```python
from build123d import *

# Parameters (mm, degrees)
BOSS_EXTRUDE1_DEPTH = 3
SKETCH1_9_R         = 1.5
SKETCH1_9_W         = 3
SKETCH1_9_H         = 3.9
SKETCH1_9_W_2       = 7.8
SKETCH1_9_H_2       = 3
BOSS_EXTRUDE2_DEPTH = 27
SKETCH2_W           = 22
SKETCH2_H           = 3.9
BOSS_EXTRUDE3_DEPTH = 2.5
CUT_EXTRUDE1_REACH  = 183.139
SKETCH6_R           = 1.95
SKETCH1_12_R        = 1.6
CUT_EXTRUDE7_DEPTH  = 105.877309271
SKETCH7_R           = 5
CUT_EXTRUDE8_DEPTH  = 10
FILLET1_R           = 3
FILLET2_R           = 3
CUT_EXTRUDE9_START  = -7.3
SKETCH8_W           = 11.4
SKETCH8_H           = 17.4
CUT_EXTRUDE9_DEPTH  = 33.4


with BuildPart() as part:
    # Sketch1 → Boss-Extrude1 (new body)
    with BuildSketch(Plane(origin=(0, 0, 0), x_dir=(1, 0, 0), z_dir=(0, 1, 0))):
        with BuildLine():
            ThreePointArc((-92, -22.5), (-86.142135624, -36.642135624), (-72, -42.5))
            Line((-72, -42.5), (72, -42.5))
            ThreePointArc((72, -42.5), (86.142135624, -36.642135624), (92, -22.5))
            Line((92, -22.5), (92, 34.5))
            Line((92, 34.5), (50, 34.5))
            Line((50, 34.5), (50, 42.5))
            Line((50, 42.5), (-50, 42.5))
            Line((-50, 42.5), (-50, 34.5))
            Line((-50, 34.5), (-92, 34.5))
            Line((-92, 34.5), (-92, -22.5))
        make_face()
    extrude(amount=BOSS_EXTRUDE1_DEPTH)

    # Sketch1<9> → Boss-Extrude2 (add)
    # profile 1 of 13: a face of its own
    with BuildSketch(Plane(origin=(0, 0, 0), x_dir=(1, 0, 0), z_dir=(0, 1, 0))):
        with BuildLine():
            ThreePointArc((-92, -22.5), (-86.142135624, -36.642135624), (-72, -42.5))
            Line((-72, -42.5), (72, -42.5))
            ThreePointArc((72, -42.5), (86.142135624, -36.642135624), (92, -22.5))
            Line((92, -22.5), (92, 34.5))
            Line((92, 34.5), (50, 34.5))
            Line((50, 34.5), (50, 42.5))
            Line((50, 42.5), (-50, 42.5))
            Line((-50, 42.5), (-50, 34.5))
            Line((-50, 34.5), (-92, 34.5))
            Line((-92, 34.5), (-92, -22.5))
        make_face()
        with Locations(Location((0, -39.5, 0), (0, 0, 270))):
            Circle(SKETCH1_9_R, mode=Mode.SUBTRACT)
        with Locations(Location((-89, 31.5, 0), (0, 0, 270))):
            Circle(SKETCH1_9_R, mode=Mode.SUBTRACT)
        with Locations(Location((-47, 39.5, 0), (0, 0, 270))):
            Circle(SKETCH1_9_R, mode=Mode.SUBTRACT)
        Polygon((-72, -36.5), (-86, -36.5), (-86, -22.5), (-86, 28.5), (-44, 28.5), (-44, 36.5), (44, 36.5), (44, 28.5), (86, 28.5), (86, -22.5), (86, -36.5), (72, -36.5), align=None, mode=Mode.SUBTRACT)
        with Locations(Location((89, 31.5, 0), (0, 0, 270))):
            Circle(SKETCH1_9_R, mode=Mode.SUBTRACT)
        with Locations(Location((47, 39.5, 0), (0, 0, 270))):
            Circle(SKETCH1_9_R, mode=Mode.SUBTRACT)
    # profile 2 of 13: a face of its own
    with BuildSketch(Plane(origin=(0, 0, 0), x_dir=(1, 0, 0), z_dir=(0, 1, 0))):
        Polygon((-57, 19.75), (-54, 19.75), (-54, 22.75), (-61.8, 22.75), (-61.8, 19.75), align=None)
    # profile 3 of 13: a face of its own
    with BuildSketch(Plane(origin=(0, 0, 0), x_dir=(1, 0, 0), z_dir=(0, 1, 0))):
        with Locations((-55.5, 17.8)):
            Rectangle(SKETCH1_9_W, SKETCH1_9_H)
    # profile 4 of 13: a face of its own
    with BuildSketch(Plane(origin=(0, 0, 0), x_dir=(1, 0, 0), z_dir=(0, 1, 0))):
        Polygon((-54, 12.85), (-54, 15.85), (-57, 15.85), (-79, 15.85), (-79, 12.85), align=None)
    # profile 5 of 13: a face of its own
    with BuildSketch(Plane(origin=(0, 0, 0), x_dir=(1, 0, 0), z_dir=(0, 1, 0))):
        Polygon((-82, 19.75), (-79, 19.75), (-74.2, 19.75), (-74.2, 22.75), (-82, 22.75), align=None)
    # profile 6 of 13: a face of its own
    with BuildSketch(Plane(origin=(0, 0, 0), x_dir=(1, 0, 0), z_dir=(0, 1, 0))):
        Polygon((-79, 12.85), (-79, 15.85), (-79, 19.75), (-82, 19.75), (-82, 12.85), align=None)
    # profile 7 of 13: a face of its own
    with BuildSketch(Plane(origin=(0, 0, 0), x_dir=(1, 0, 0), z_dir=(0, 1, 0))):
        with Locations((57.9, 21.25)):
            Rectangle(SKETCH1_9_W_2, SKETCH1_9_H_2)
    # profile 8 of 13: a face of its own
    with BuildSketch(Plane(origin=(0, 0, 0), x_dir=(1, 0, 0), z_dir=(0, 1, 0))):
        with Locations((55.5, 17.8)):
            Rectangle(SKETCH1_9_W, SKETCH1_9_H)
    # profile 9 of 13: a face of its own
    with BuildSketch(Plane(origin=(0, 0, 0), x_dir=(1, 0, 0), z_dir=(0, 1, 0))):
        Polygon((79, 15.85), (57, 15.85), (54, 15.85), (54, 12.85), (79, 12.85), align=None)
    # profile 10 of 13: a face of its own
    with BuildSketch(Plane(origin=(0, 0, 0), x_dir=(1, 0, 0), z_dir=(0, 1, 0))):
        with Locations((78.1, 21.25)):
            Rectangle(SKETCH1_9_W_2, SKETCH1_9_H_2)
    # profile 11 of 13: a face of its own
    with BuildSketch(Plane(origin=(0, 0, 0), x_dir=(1, 0, 0), z_dir=(0, 1, 0))):
        Polygon((79, 19.75), (79, 15.85), (79, 12.85), (82, 12.85), (82, 19.75), align=None)
    # profile 12 of 13: a face of its own
    with BuildSketch(Plane(origin=(0, 0, 0), x_dir=(1, 0, 0), z_dir=(0, 1, 0))):
        with BuildLine():
            Line((-86, -22.5), (-86, -36.5))
            Line((-86, -36.5), (-72, -36.5))
            ThreePointArc((-72, -36.5), (-81.899494937, -32.399494937), (-86, -22.5))
        make_face()
        with Locations(Location((-84.02081528, -34.52081528, 0), (0, 0, 270))):
            Circle(SKETCH1_9_R, mode=Mode.SUBTRACT)
    # profile 13 of 13: a face of its own
    with BuildSketch(Plane(origin=(0, 0, 0), x_dir=(1, 0, 0), z_dir=(0, 1, 0))):
        with BuildLine():
            ThreePointArc((86, -22.5), (81.899494937, -32.399494937), (72, -36.5))
            Line((72, -36.5), (86, -36.5))
            Line((86, -36.5), (86, -22.5))
        make_face()
        with Locations(Location((84.02081528, -34.52081528, 0), (0, 0, 270))):
            Circle(SKETCH1_9_R, mode=Mode.SUBTRACT)
    extrude(amount=BOSS_EXTRUDE2_DEPTH)

    # Sketch2 → Boss-Extrude3 (add)
    with BuildSketch(Plane(origin=(0, 3, 0), x_dir=(1, 0, 0), z_dir=(0, 1, 0))):
        with Locations((-68, 17.8)):
            Rectangle(SKETCH2_W, SKETCH2_H)
        with Locations((68, 17.8)):
            Rectangle(SKETCH2_W, SKETCH2_H)
    extrude(amount=BOSS_EXTRUDE3_DEPTH)

    # Cut-Extrude1: up to this face of the body (flat: up to its plane)
    cut_extrude1_end = Plane(part.part.faces().sort_by_distance((82, 15, -17.8))[0])
    # Sketch6 → Cut-Extrude1 (cut, up to the picked face)
    with BuildSketch(Plane.ZY.offset(82), mode=Mode.PRIVATE) as cut_extrude1_sk1:
        with Locations((-17.8, 16.5)):
            Circle(SKETCH6_R)
    cut_extrude1_tool1 = split(extrude(cut_extrude1_sk1.sketch, amount=-CUT_EXTRUDE1_REACH, mode=Mode.PRIVATE), bisect_by=cut_extrude1_end, keep=Keep.BOTH, mode=Mode.PRIVATE)
    add(cut_extrude1_tool1.solids().sort_by(Axis((-82, 16.5, -17.8), (1, 0, 0)))[0], mode=Mode.SUBTRACT)

    # Sketch1<12> → Cut-Extrude7 (cut, through all)
    with BuildSketch(Plane(origin=(0, 0, 0), x_dir=(1, 0, 0), z_dir=(0, 1, 0))):
        with Locations(Location((-64.4, -13.9, 0), (0, 0, 270))):
            Circle(SKETCH1_12_R)
        with Locations(Location((-37.6, -13.9, 0), (0, 0, 270))):
            Circle(SKETCH1_12_R)
        with Locations(Location((64.4, 5.9, 0), (0, 0, 270))):
            Circle(SKETCH1_12_R)
        with Locations(Location((37.6, 5.9, 0), (0, 0, 270))):
            Circle(SKETCH1_12_R)
        with Locations(Location((64.4, -13.9, 0), (0, 0, 270))):
            Circle(SKETCH1_12_R)
        with Locations(Location((37.6, -13.9, 0), (0, 0, 270))):
            Circle(SKETCH1_12_R)
        with Locations(Location((-64.4, 5.9, 0), (0, 0, 270))):
            Circle(SKETCH1_12_R)
        with Locations(Location((-37.6, 5.9, 0), (0, 0, 270))):
            Circle(SKETCH1_12_R)
    extrude(amount=CUT_EXTRUDE7_DEPTH, mode=Mode.SUBTRACT)

    # Sketch7 → Cut-Extrude8 (cut)
    with BuildSketch(Plane(origin=(0, 0, -42.5), x_dir=(-1, 0, 0), z_dir=(0, 0, -1))):
        with Locations((0, 15)):
            Circle(SKETCH7_R)
    extrude(amount=-CUT_EXTRUDE8_DEPTH, mode=Mode.SUBTRACT)

    # Fillet1
    fillet1_edges = [part.edges().sort_by_distance(p)[0] for p in [
        (-86, 15, -28.5),
        (-44, 15, -28.5),
        (-44, 15, -36.5),
        (44, 15, -36.5),
        (44, 15, -28.5),
        (-92, 13.5, -34.5),
        (-50, 13.5, -34.5),
        (-50, 13.5, -42.5),
        (50, 13.5, -42.5),
        (50, 13.5, -34.5),
        (92, 13.5, -34.5),
    ]]
    fillet(fillet1_edges, radius=FILLET1_R)

    # Fillet2
    fillet2_edges = [part.edges().sort_by_distance(p)[0] for p in [
        (54, 15, -22.75),
        (54, 15, -12.85),
        (82, 15, -12.85),
        (82, 15, -22.75),
        (-82, 15, -22.75),
        (-82, 15, -12.85),
        (-54, 15, -12.85),
        (-54, 15, -22.75),
    ]]
    fillet(fillet2_edges, radius=FILLET2_R - 0.0001)  # a hair under: the kernel refuses the full size

    # Sketch8 → Cut-Extrude9 (cut)
    with BuildSketch(Plane.ZY.offset(92).offset(CUT_EXTRUDE9_START)):
        with Locations((-31.1, 16.5)):
            Rectangle(SKETCH8_W, SKETCH8_H)
    cut_extrude9 = extrude(amount=-CUT_EXTRUDE9_DEPTH, mode=Mode.SUBTRACT)

    # Mirror1: Cut-Extrude9 across plane
    add(cut_extrude9.mirror(Plane(origin=(0, 0, 0), x_dir=(0, 0, 1), z_dir=(1, 0, 0))), mode=Mode.SUBTRACT)


solid = part.part
```
Work out the finished part from the listing and answer in its coordinate system (mm). A direction names the side the tool comes from. Round coordinates to 2 decimals unless told otherwise and drop trailing zeros. Write each loop counter-clockwise with the first axis right and the second up, starting at its lowest first coordinate (ties: lowest second). Pieces come first, ordered by that corner, then holes. Notation, with made-up numbers: (42.25, -13.5) -> (51.25, -13.5) arc R23 ccw to (51.25, 10.5) -> close; hole circle Ø10 at (11.5, 60). An arc over 180 degrees is marked (long way). Write each question's results on one line, items separated by ' | '.
Q1. Determine the mould class of faces 5 (the flat face through (79, 10, -18)), 6 (the flat face through (67.8, 27, -15.7)), 7 (the cylindrical face through (1.08, 10.12, -39.54)) for opening direction Y: released by +Y, released by -Y, zero draft, split by the parting line, or undercut.
Data:
face 5: zero draft | face 6: released by +Y | face 7: undercut
Q2. Flat-ended cylindrical pins translate along their axes: P1, Ø6, axis at x = -58, y = 5.5, coming from the -Z side; P2, Ø2.5, axis at x = 89, z = -31.5, coming from the +Y side. Find the tip coordinate at first contact, or state that the pin passes through.
Data:
P1: z = -34.5 | P2: y = 3
Q3. Section B-B, the plane y = 12.5 is taken. Give the number of separate pieces and of enclosed holes in the cut face, then the cut area to 3 significant figures.
Data:
separate pieces: 5 | enclosed holes: 7 | area: 2,780 mm^2
Q4. Straight lines are drawn through the part: line 1 along X through (y, z) = (13.25, -31.5); line 2 along X through (y, z) = (10, -18.5); line 3 along X through (y, z) = (2.05, 13.9). For each, find the intervals that lie inside material, in ascending order. Write a range as [from, to].
Data:
line 1: [-92, -90.5], [-87.5, -84.7], [-51.3, -44], [44, 51.3], [84.7, 87.5], [90.5, 92] | line 2: [-92, -86], [-82, -79], [-57, -54], [54, 57], [79, 82], [86, 92] | line 3: [-92, -66], [-62.8, -39.2], [-36, 36], [39.2, 62.8], [66, 92]
Q5. Which of the six approach directions +Z, -Z, +X, -X, +Y, -Y give full straight-line access (tool end or side, diameter ignored) to faces 1 (the flat face through (-0.4, 27, 37.6)), 2 (the flat face through (-68, 25.2, -32)), 3 (the flat face through (77, 15, -22.75)), 4 (the cylindrical face through (80.479, 14.596, -18.223))?
Data:
face 1: +Z, -Z, +X, -X, +Y | face 2: -Z | face 3: +Y | face 4: none
Q6. Section A-A, the plane x = -29 is taken. Write down the section's boundary in (y, z), then the cut area to 3 significant figures.
Data:
outline: (0, -42.5) -> (27, -42.5) -> (27, -36.5) -> (3, -36.5) -> (3, 36.5) -> (27, 36.5) -> (27, 42.5) -> (0, 42.5) -> close | area: 543 mm^2
